The listing builds one solid part. Answer for the finished solid, in the listing's coordinates (mm). Round coordinates to 2 decimals unless told otherwise and drop trailing zeros. Loops run counter-clockwise (first coordinate to the right, second up) from the corner with the lowest first, then second, coordinate; pieces in that order, holes last. Notation, with made-up numbers: (30.25, 24.5) -> (60.25, 24.5) arc R4 cw to (60.25, 28.5) -> close; hole circle Ø8 at (-27.5, 2.5). An arc over 180 degrees is marked (long way). Answer in a Markdown table with one row per item. Add a question column.
```python
from build123d import *

# Parameters (mm, degrees)
F0_W     = 17.5
F0_H     = 17.5
F1_DEPTH = 8.75
F2_SIZE  = 2


with BuildPart() as f1:
    # F0 (on Top) → F1 (new body, symmetric)
    with BuildSketch(Plane.XY):
        Rectangle(F0_W, F0_H)
    extrude(amount=F1_DEPTH, both=True)

    # F2
    f2_edges = [f1.edges().sort_by_distance(p)[0] for p in [
        (-8.75, 0, 8.75),
        (0, -8.75, 8.75),
        (8.75, 0, 8.75),
        (0, 8.75, 8.75),
        (8.75, -8.75, 0),
        (8.75, 8.75, 0),
        (8.75, 0, -8.75),
        (0, 8.75, -8.75),
        (-8.75, 8.75, 0),
        (-8.75, -8.75, 0),
        (0, -8.75, -8.75),
        (-8.75, 0, -8.75),
    ]]
    chamfer(f2_edges, length=F2_SIZE)


solid = f1.part
```
Item 1: Section A-A, the plane y = -2.75 is taken. Write down the section's boundary in (x, z).
Item 2: Consider L1, parallel to X at y = 8, z = 3.5; L2, parallel to X at y = -3, z = 7; L3, parallel to Z at x = -6.5, y = -7.75. Determine where each line is inside the solid, lowest interval first. Write a range as from..to.
Here are the results:
| question | item | result |
|---|---|---|
| 1 | outline | (-8.75, -6.75) -> (-6.75, -8.75) -> (6.75, -8.75) -> (8.75, -6.75) -> (8.75, 6.75) -> (6.75, 8.75) -> (-6.75, 8.75) -> (-8.75, 6.75) -> close |
| 2 | L1 | x = -7.5..7.5 |
| 2 | L2 | x = -8.5..8.5 |
| 2 | L3 | z = -7.75..7.75 |
